Study the drawing (mm; zero at the part's minimum x, y, z) and answer. A direction names the side the tool comes from. Give positions to 0.01 mm unless a question says otherwise; leave off trailing zeros. Write each loop counter-clockwise with the first axis right and the second up, starting at its lowest first coordinate (ties: lowest second). Pieces come first, ordered by that corner, then holes. Notation, with made-up numbers: (58, -12) - (92, -12) arc R18 cw to (92, 12) - close; hole circle Ø6 at (-18.75, -20.5). An arc over 180 degrees is marked (long way). Return JSON: item names as keys, results as strings.
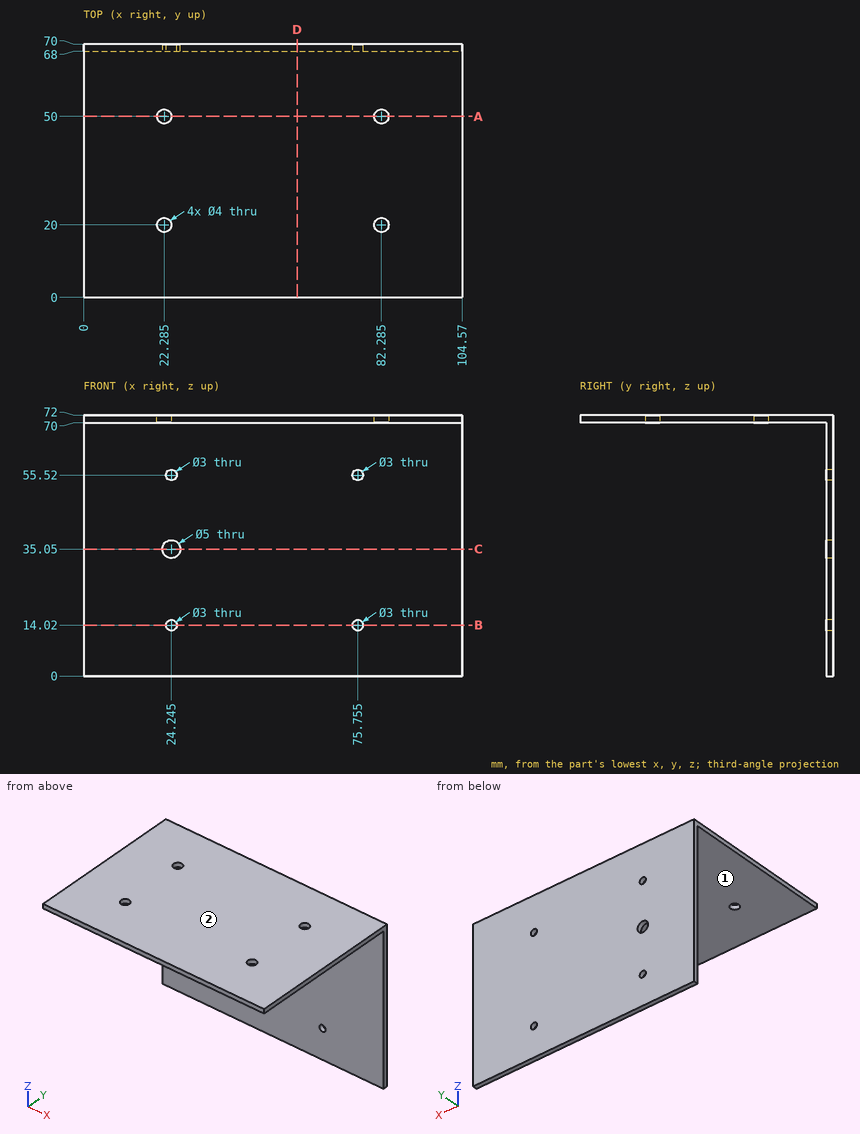
Item 1: For the marked faces 1 and 2, determine the directions among +Z, -Z, +X, -X, +Y, -Y from which every point of the face is accessible in a straight line to the end or side of a thin tool.
Answer below:
{"face 1": "-Z, +X, -X, -Y", "face 2": "+Z, +X, -X, +Y, -Y"}
Item 2: Consider L1, parallel to X at y = 69.25, z = 14.02 (3 decimals); L2, parallel to Y at x = 27, z = 56.5; L3, parallel to Z at x = 46, y = 4. Determine where each line is inside the solid, lowest interval first.
Answer below:
{"L1": "x = 0 to 22.745, 25.745 to 74.255, 77.255 to 104.57", "L2": "y = 68 to 70", "L3": "z = 70 to 72"}
Item 3: A cutting plane is placed at D-D on x = 59. Determine the outline of the cut face in (y, z), then the cut area to 3 significant figures.
Answer below:
{"outline": "(0, 70) - (68, 70) - (68, 0) - (70, 0) - (70, 72) - (0, 72) - close", "area": "280 mm²"}
Item 4: A cutting plane is placed at B-B on z = 14.02. Determine the outline of the cut face in (x, y) (3 decimals), then the cut area to 3 significant figures.
Answer below:
{"outline": "(0, 68) - (22.745, 68) - (22.745, 70) - (0, 70) - close; (25.745, 68) - (74.255, 68) - (74.255, 70) - (25.745, 70) - close; (77.255, 68) - (104.57, 68) - (104.57, 70) - (77.255, 70) - close", "area": "197 mm²"}
Item 5: Flat-ended cylindrical pins translate along their axes: P1, Ø6.5, axis at x = 24.245, z = 35.05, coming from the -Y side; P2, Ø6.5, axis at x = 22.285, y = 50, coming from the +Z side; P3, Ø4, axis at x = 50, y = 47.5, coming from the -Z side. Find the tip coordinate at first contact, or state that the pin passes through.
Answer below:
{"P1": "stops at y = 68", "P2": "stops at z = 72", "P3": "stops at z = 70"}
Item 6: A cutting plane is placed at A-A on y = 50. Determine the outline of the cut face in (x, z) (3 decimals).
Answer below:
{"outline": "(0, 70) - (20.285, 70) - (20.285, 72) - (0, 72) - close; (24.285, 70) - (80.285, 70) - (80.285, 72) - (24.285, 72) - close; (84.285, 70) - (104.57, 70) - (104.57, 72) - (84.285, 72) - close"}
Item 7: A cutting plane is placed at C-C on z = 35.05. Determine the outline of the cut face in (x, y) (3 decimals).
Answer below:
{"outline": "(0, 68) - (21.745, 68) - (21.745, 70) - (0, 70) - close; (26.745, 68) - (104.57, 68) - (104.57, 70) - (26.745, 70) - close"}
